```python
from build123d import *

# Parameters (mm, degrees)
BOSS_EXTRUDE2_DEPTH  = 50
BOSS_EXTRUDE10_DEPTH = 1.5
BOSS_EXTRUDE11_DEPTH = 1.5


with BuildPart() as part:
    # Sketch1 → Boss-Extrude2 (new body)
    with BuildSketch(Plane(origin=(0, 0, 0), x_dir=(0, 0, -1), z_dir=(1, 0, 0))):
        Polygon((0, 7.671680622), (0, 0), (2, 0), (2, 13.6), (30, 13.6), (30, 15.1), (2, 15.1), (2, 19), (30, 19), (30, 20), (0, 20), (0, 12.5), (-1.7, 12.5), (-1.7, 15.25), (-4.45, 12.5), (-4.45, 7.671680622), (-1.7, 4.921680622), (-1.7, 7.671680622), align=None)
    extrude(amount=BOSS_EXTRUDE2_DEPTH)

    # Sketch1_13 → Boss-Extrude10 (add)
    with BuildSketch(Plane(origin=(0, 0, 0), x_dir=(0, 0, -1), z_dir=(1, 0, 0))):
        Polygon((30, 13.6), (2, 0), (2, 13.6), align=None)
    extrude(amount=BOSS_EXTRUDE10_DEPTH)

    # Sketch7 → Boss-Extrude11 (add)
    with BuildSketch(Plane(origin=(50, 0, 0), x_dir=(0, 0, -1), z_dir=(1, 0, 0))):
        Polygon((2, 13.6), (2, 0), (30, 13.6), align=None)
    extrude(amount=-BOSS_EXTRUDE11_DEPTH)


solid = part.part
```
Could you check a few things on this model? Use its own coordinates, in mm. A direction names the side the tool comes from. Give positions to 0.01 mm unless a question says otherwise; leave off trailing zeros. Order: outer loops, then holes, each group sorted by start corner. A loop starts at its lowest first (then second) coordinate and runs counter-clockwise, first axis right, second up.
Q1. Suppose I cut it at C-C, the plane y = 6.25. Write out the boundary of the cut face in (x, z), and give its area (3 significant figures).
Q2. For faces 5 (the flat face through (25, 19, -16)), 6 (the flat face through (25, 7, -2)), 7 (the flat face through (25, 14, -30)), 8 (the flat face through (25, 6, 1.7)), 9 (the flat face through (25, 16, 0)), which set-ups out of +Z, -Z, +X, -X, +Y, -Y let a thin tool reach every point of the face, with its end or its side?
Q3. I'm going to push flat-ended pins straight in: P1, Ø4, axis at x = 22, y = 3, coming from the +Z side; P2, Ø0.5, axis at x = 30.5, z = 1, coming from the -Y side; P3, Ø1.2, axis at x = 24, y = 17, coming from the -Z side. Where does each tip first touch, or does it pass through?
Q4. We'd pull the mould along X, two halves only. Please class faces 1 (the flat face through (0, 12, -9)), 2 (the flat face through (48.5, 8, -13)), 3 (the flat face through (24.6, 19.5, -30)), 4 (the flat face through (25, 13.6, -16)): +X half, -X half, draft (parallel to the pull), parting line (faces both ways), or undercut.
Q5. Suppose I cut it at B-B, the plane x = 29. Write out the boundary of the cut face in (y, z), and give its area (3 significant figures).
Q6. Suppose I cut it at D-D, the plane y = 2.25. Write out the boundary of the cut face in (x, z), and give its area (3 significant figures).
Q7. Suppose I cut it at A-A, the plane z = -19.5. Write out the boundary of the cut face in (x, y), and give its area (3 significant figures).
Q8. If I drill on line 1 along Y through (x, z) = (38, -24.5); line 2 along X through (y, z) = (13, -24.5); line 3 along Z through (x, y) = (17, 5.25), over which ranges is the centre line in solid material (lowest first)?
Solution:
1. outline: (0, -14.87) - (1.5, -14.87) - (1.5, -2) - (48.5, -2) - (48.5, -14.87) - (50, -14.87) - (50, 0) - (0, 0) - close; (0, 1.7) - (50, 1.7) - (50, 3.03) - (0, 3.03) - close
1. area: 205 mm2
2. face 5: -Z, +X, -X
2. face 6: -Z, -Y
2. face 7: -Z, +X, -X, +Y, -Y
2. face 8: +X, -X, -Y
2. face 9: +X, -X, +Y
3. P1: stops at z = 1.78
3. P2: stops at y = 7.67
3. P3: stops at z = -2
4. face 1: -X half
4. face 2: undercut
4. face 3: draft
4. face 4: undercut
5. outline: (0, -2) - (13.6, -2) - (13.6, -30) - (15.1, -30) - (15.1, -2) - (19, -2) - (19, -30) - (20, -30) - (20, 0) - (12.5, 0) - (12.5, 1.7) - (15.25, 1.7) - (12.5, 4.45) - (7.67, 4.45) - (4.92, 1.7) - (7.67, 1.7) - (7.67, 0) - (0, 0) - close
5. area: 139 mm2
6. outline: (0, -6.63) - (1.5, -6.63) - (1.5, -2) - (48.5, -2) - (48.5, -6.63) - (50, -6.63) - (50, 0) - (0, 0) - close
6. area: 114 mm2
7. outline: (0, 8.5) - (1.5, 8.5) - (1.5, 13.6) - (48.5, 13.6) - (48.5, 8.5) - (50, 8.5) - (50, 15.1) - (0, 15.1) - close; (0, 19) - (50, 19) - (50, 20) - (0, 20) - close
7. area: 140 mm2
8. line 1: y = 13.6 to 15.1, 19 to 20
8. line 2: x = 0 to 1.5, 48.5 to 50
8. line 3: z = -2 to 0, 1.7 to 2.03
